Autodesk Inventor part; units mm, degrees
ref_plane "YZ Plane" through (0, 0, 0) normal (1, 0, 0) x (0, 1, 0)
ref_plane "XZ Plane" through (0, 0, 0) normal (0, 1, 0) x (-1, 0, 0)
ref_plane "XY Plane" through (0, 0, 0) normal (0, 0, 1) x (1, 0, 0)
sketch "Sketch1" plane through (0, 0, 0) normal (0, 1, 0) x (-1, 0, 0)
  line L0 (25.4, 60.325) -> (-25.4, 60.325)
  line L1 (-25.4, 60.325) -> (-25.4, -60.325)
  line L2 (-25.4, -60.325) -> (25.4, -60.325)
  line L3 (25.4, -60.325) -> (25.4, 60.325)
  line L4 (25.4, 60.325) -> (-25.4, -60.325) construction
  line L5 (-25.4, 60.325) -> (25.4, -60.325) construction
  point P0 (0, 0)
  point P1 (0, 28.575)
  point P2 (0, -28.575)
  dimension "d0" = 50.8
  dimension "d1" = 120.65
  dimension "d2" = 57.15
  dimension "d3" = 28.575
extrude "Plate1" add sketch "Sketch1" along normal blind 6.35
sketch "Sketch2" plane through (0, 0, 0) normal (0, -1, 0) x (1, 0, 0)
  circle A0 centre (0, 28.575) radius 5.715
  circle A1 centre (0, -28.575) radius 4.1
  point P0 (0, 0)
  dimension "d5" = 28.575
  dimension "d6" = 11.43
  dimension "d9" = 28.575
  dimension "d10" = 8.2
extrude "Cut1" cut sketch "Sketch2" against normal blind 6.35
sketch "Sketch3" plane through (0, 0, 0) normal (0, -1, 0) x (1, 0, 0)
  line L0 (-25.4, 60.325) -> (25.4, 60.325) construction
  line L1 (-25.4, -60.325) -> (-25.4, 60.325) construction
  circle A0 centre (0, 28.575) radius 5.715
  circle A1 centre (0, 28.575) radius 25.4 construction
  circle A2 centre (0, -28.575) radius 4.1
  circle A3 centre (0, -28.575) radius 25.4 construction
  point P0 (0, 0)
  point P1 (-19.05, 53.975)
  point P2 (19.05, 53.975)
  point P3 (-19.05, 0)
  point P4 (19.05, 0)
  point P5 (-19.05, -53.975)
  point P6 (19.05, -53.975)
  dimension "d13" = 38.1
  dimension "d16" = 53.975
  dimension "d19" = 6.35
  dimension "d20" = 6.35
  dimension "d29" = 50.8
  dimension "d30" = 50.8
hole "Hole1" at (-19.05, 0, 53.975) at (19.05, 0, 53.975) at (-19.05, 0, 0) at (19.05, 0, 0) at (-19.05, 0, -53.975) at (19.05, 0, -53.975) direction (0, 1, 0) diameter 5.1054 end through all
fillet "Corner Round1" radius 6.35 4 edges at (25.4, 3.175, -60.325) (-25.4, 3.175, -60.325) (25.4, 3.175, 60.325) (-25.4, 3.175, 60.325)
equation "\"d7\" = Thickness"
equation "\"d26\" = Thickness"
equation "\"d4\" = Thickness"
equation "\"BendRadius\" = Thickness"
equation "\"BendReliefWidth\" = Thickness"
equation "\"BendReliefDepth\" = 0.5 * Thickness"
equation "\"CornerReliefSize\" = 4 * Thickness"
equation "\"MinimumRemnant\" = 2 * Thickness"
equation "\"TransitionRadius\" = BendRadius"
equation "\"JacobiRadiusSize\" = BendRadius"
equation "\"GapSize\" = Thickness"
properties part number "PLATE,MAGNET-MOUNT" material "Aluminum 6061"
Verification items for the finished model (mm, model axes). Give positions to 0.01 mm unless a question says otherwise; leave off trailing zeros. Order: outer loops, then holes, each group sorted by start corner. A loop starts at its lowest first (then second) coordinate and runs counter-clockwise, first axis right, second up. Notation, with made-up numbers: M 52.25,36 L 70.25,36 A26 ccw 70.25,69 Z; hole C -1,-5 d3. An arc over 180 degrees is marked long. Answer in a Markdown table with one row per item. Add a question column.
Item 1: Section check B-B, the plane x = 0. Enter the section's corners in (y, z) (3 decimals), and give its area (3 significant figures).
Item 2: Mould release check, pull along X, two halves, no side actions. Record for faces 1 (the cylindrical face through (-18.07, 3.22, -56.33)), 2 (the cylindrical face through (16.898, 3.219, -1.372)), 3 (the cylindrical face through (23.49, 3.219, 58.514)), 4 (the flat face through (0, 3, -60.325)): released by +X, released by -X, zero draft, split by the parting line, or undercut.
Item 3: Scan lines: probe 1 along Z at (x, y) = (19.05, 2.25) (3 decimals); probe 2 along X at (y, z) = (5.25, 0); probe 3 along Z at (x, y) = (0, 2.5) (3 decimals). Record each from-to range of solid material in increasing order. Write a range as from..to.
Item 4: Section check A-A, the plane z = 0. Enter the section's corners in (x, y).
Item 5: Section check C-C, the plane y = 2.5. State how many separate pieces and enclosed holes the cut face has, and give its area (3 significant figures).
Filled sheet:
| question | item | result |
|---|---|---|
| 1 | outline | M 0,-60.325 L 6.35,-60.325 L 6.35,-32.675 L 0,-32.675 Z; M 0,-24.475 L 6.35,-24.475 L 6.35,22.86 L 0,22.86 Z; M 0,34.29 L 6.35,34.29 L 6.35,60.325 L 0,60.325 Z |
| 1 | area | 641 mm^2 |
| 2 | face 1 | undercut |
| 2 | face 2 | undercut |
| 2 | face 3 | released by +X |
| 2 | face 4 | zero draft |
| 3 | probe 1 | z = -60.325..-56.528, -51.422..-2.553, 2.553..51.422, 56.528..60.325 |
| 3 | probe 2 | x = -25.4..-21.6, -16.5..16.5, 21.6..25.4 |
| 3 | probe 3 | z = -60.325..-32.675, -24.475..22.86, 34.29..60.325 |
| 4 | outline | M -25.4,0 L -21.6,0 L -21.6,6.35 L -25.4,6.35 Z; M -16.5,0 L 16.5,0 L 16.5,6.35 L -16.5,6.35 Z; M 21.6,0 L 25.4,0 L 25.4,6.35 L 21.6,6.35 Z |
| 5 | separate pieces | 1 |
| 5 | enclosed holes | 8 |
| 5 | area | 5,820 mm^2 |
